Drawing for the job (mm, zero at the part's lowest x, y, z). Give positions to 0.01 mm unless a question says otherwise; leave off trailing zeros. Order: outer loops, then holes, each group sorted by start corner. A loop starts at its lowest first (then second) coordinate and runs counter-clockwise, first axis right, second up. Notation, with made-up numbers: (-2.5, 54) - (53.5, 54) arc R21 ccw to (53.5, 72) - close; hole circle Ø9 at (-6.5, 5.25). An arc over 180 degrees is marked (long way). One line per item, written item: value.
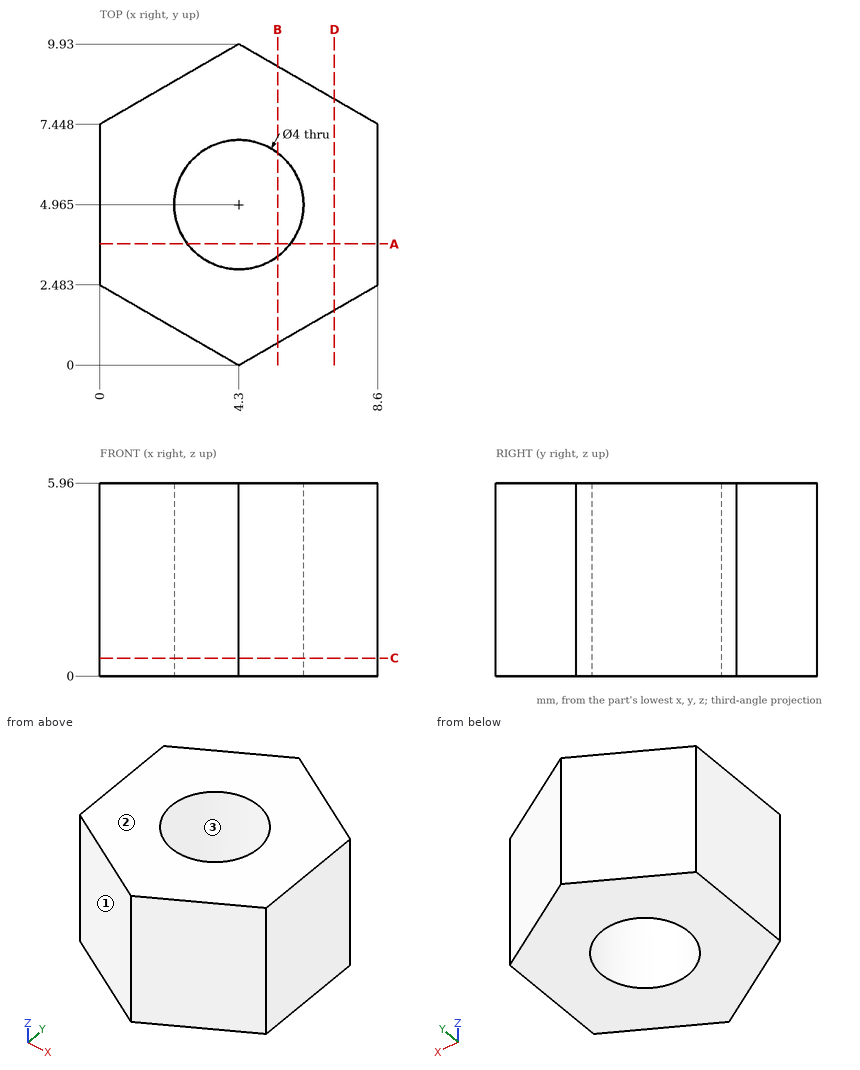
(1) Slice it at D-D, the plane x = 7.25. Give the cut face in (y, z), and give its area (3 significant figures).
Completed:
outline: (1.7, 0) - (8.23, 0) - (8.23, 5.96) - (1.7, 5.96) - close
area: 38.9 mm²
(2) Drill centre lines: line 1 (X direction, y = 5, z = 5); line 2 (X direction, y = 4.5, z = 2.5) (1 decimal); line 3 (Y direction, x = 5.5, z = 4.5) (1 decimal). Where is each one in solid material? Low to high.
Completed:
line 1: 0 to 2.3, 6.3 to 8.6
line 2: 0 to 2.4, 6.2 to 8.6
line 3: 0.7 to 3.4, 6.6 to 9.2
(3) Slice it at B-B, the plane x = 5.5. Give the cut face in (y, z) (1 decimal).
Completed:
outline: (0.7, 0) - (3.4, 0) - (3.4, 6) - (0.7, 6) - close; (6.6, 0) - (9.2, 0) - (9.2, 6) - (6.6, 6) - close
(4) Pull direction Y, two halves, no side cores. Call the marked faces 1, 2 and 3: +Y half, -Y half, draft (parallel to the pull), parting line (faces both ways), or undercut.
Completed:
face 1: -Y half
face 2: draft
face 3: undercut
(5) Slice it at C-C, the plane z = 0.55. Give the cut face in (x, y) (1 decimal).
Completed:
outline: (0, 2.5) - (4.3, 0) - (8.6, 2.5) - (8.6, 7.4) - (4.3, 9.9) - (0, 7.4) - close; hole circle Ø4 at (4.3, 5)
(6) Slice it at A-A, the plane y = 3.75. Give the cut face in (x, z).
Completed:
outline: (0, 0) - (2.71, 0) - (2.71, 5.96) - (0, 5.96) - close; (5.89, 0) - (8.6, 0) - (8.6, 5.96) - (5.89, 5.96) - close
